Verification items for the finished model (mm, model axes). Round coordinates to 2 decimals unless told otherwise and drop trailing zeros. Order: outer loops, then holes, each group sorted by start corner. A loop starts at its lowest first (then second) coordinate and runs counter-clockwise, first axis right, second up. Notation, with made-up numbers: (-4.5, 32) -> (18.5, 32) arc R23 cw to (18.5, 48) -> close; hole circle Ø5 at (-35.75, 28). An arc over 180 degrees is marked (long way). Put each result on its own line as item: value.
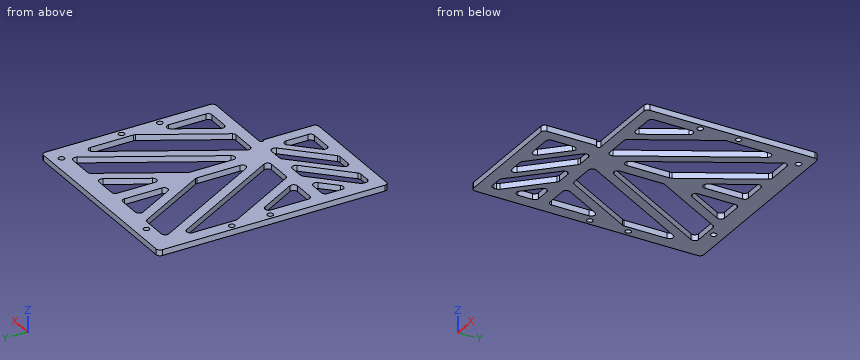
```python
from build123d import *

# Parameters (mm, degrees)
SKETCH_1_W          = 103.5
SKETCH_1_H          = 90
EXTRUDE_1_DEPTH     = 1.5
SKETCH_2_W          = 63.5
SKETCH_2_H          = 30
EXTRUDE_2_DEPTH     = 3
SKETCH_3_R          = 1.05
CUT_EXTRUDE_1_DEPTH = 3
SKETCH_4_R          = 1.525
CUT_EXTRUDE_2_DEPTH = 10
SKETCH_5_R          = 1.525
CUT_EXTRUDE_3_DEPTH = 10
FILLET_1_R          = 2
CUT_EXTRUDE_4_DEPTH = 10
CUT_EXTRUDE_5_DEPTH = 10
FILLET_2_R          = 2


with BuildPart() as part:
    # 草图1 → 凸台-拉伸1 (new, symmetric)
    with BuildSketch(Plane.XY):
        Rectangle(SKETCH_1_W, SKETCH_1_H)
    extrude(amount=EXTRUDE_1_DEPTH, both=True)

    # 草图2 → 凸台-拉伸2 (add)
    with BuildSketch(Plane.XY.offset(1.5)):
        with Locations((-20, -60)):
            Rectangle(SKETCH_2_W, SKETCH_2_H)
    extrude(amount=-EXTRUDE_2_DEPTH)

    # 草图3 → 切除-拉伸1 (cut)
    with BuildSketch(Plane(origin=(0, 0, -1.5), x_dir=(-1, 0, 0), z_dir=(0, 0, -1))):
        with Locations((-11.75, -46.05)):
            Circle(SKETCH_3_R)
    extrude(amount=-CUT_EXTRUDE_1_DEPTH, mode=Mode.SUBTRACT)

    # 草图4 → 切除-拉伸2 (cut)
    with BuildSketch(Plane.XY.offset(1.5)):
        with Locations((-31.749999997, 39.499993227)):
            Circle(SKETCH_4_R)
        with Locations((43.25, 39.499993227)):
            Circle(SKETCH_4_R)
    extrude(amount=-CUT_EXTRUDE_2_DEPTH, mode=Mode.SUBTRACT)

    # 草图5 → 切除-拉伸3 (cut)
    with BuildSketch(Plane(origin=(0, 0, -1.5), x_dir=(-1, 0, 0), z_dir=(0, 0, -1))):
        with Locations((48.75, -15)):
            Circle(SKETCH_5_R)
        with Locations((48.75, 5)):
            Circle(SKETCH_5_R)
    cut_extrude_3 = extrude(amount=-CUT_EXTRUDE_3_DEPTH, mode=Mode.SUBTRACT)

    # 镜向1: 切除-拉伸3 across plane
    add(cut_extrude_3.mirror(Plane(origin=(0, 0, 0), x_dir=(0, 0, 1), z_dir=(1, 0, 0))), mode=Mode.SUBTRACT)

    # 圆角1
    fillet_1_edges = [part.edges().sort_by_distance(p)[0] for p in [
        (11.75, -75, 0),
        (-51.75, -75, 0),
        (51.75, -45, 0),
        (-51.75, 45, 0),
        (51.75, 45, 0),
    ]]
    fillet(fillet_1_edges, radius=FILLET_1_R)

    # 草图6 → 切除-拉伸4 (cut)
    with BuildSketch(Plane(origin=(0, 0, -1.5), x_dir=(-1, 0, 0), z_dir=(0, 0, -1))):
        Polygon((-28.82451653, -39), (-45.25, -9.842339669), (-45.25, -39), align=None)
        Polygon((-5.869390726, -39), (-45.25, 30.906400683), (-45.25, 0.344845419), (-23.085735079, -39), align=None)
        Polygon((-25.164264921, 35.999993227), (-42.380609274, 35.999993227), (-3, -33.906407456), (-3, -3.344852192), align=None)
        Polygon((-3, 35.999993227), (-19.42548347, 35.999993227), (-3, 6.842332896), align=None)
        Polygon((3, 6.842332896), (19.42548347, 35.999993227), (3, 35.999993227), align=None)
        Polygon((42.380609274, 35.999993227), (25.164264921, 35.999993227), (3, -3.344852192), (3, -33.906407456), align=None)
        Polygon((45.25, 0.344845419), (45.25, 30.906400683), (5.869390726, -39), (23.085735079, -39), align=None)
        Polygon((45.25, -39), (45.25, -9.842339669), (28.82451653, -39), align=None)
    extrude(amount=-CUT_EXTRUDE_4_DEPTH, mode=Mode.SUBTRACT)

    # 草图7 → 切除-拉伸5 (cut)
    with BuildSketch(Plane(origin=(0, 0, -1.5), x_dir=(-1, 0, 0), z_dir=(0, 0, -1))):
        Polygon((12.593145751, -69), (-5.75, -50.656854249), (-5.75, -69), align=None)
        Polygon((6.977922061, -45), (-5.75, -45), (18.25, -69), (30.977922061, -69), align=None)
        Polygon((25.362698372, -45), (12.634776311, -45), (36.634776311, -69), (45.25, -69), (45.25, -64.887301628), align=None)
        Polygon((45.25, -45), (31.019552622, -45), (45.25, -59.230447378), align=None)
    extrude(amount=-CUT_EXTRUDE_5_DEPTH, mode=Mode.SUBTRACT)

    # 圆角2
    fillet_2_edges = [part.edges().sort_by_distance(p)[0] for p in [
        (-3, 6.842332896, 0),
        (-3, 35.999993227, 0),
        (-19.42548347, 35.999993227, 0),
        (19.42548347, 35.999993227, 0),
        (3, 35.999993227, 0),
        (3, 6.842332896, 0),
        (45.25, 0.344845419, 0),
        (45.25, 30.906400683, 0),
        (5.869390726, -39, 0),
        (23.085735079, -39, 0),
        (25.164264921, 35.999993227, 0),
        (3, -3.344852192, 0),
        (3, -33.906407456, 0),
        (42.380609274, 35.999993227, 0),
        (-45.25, -9.842339669, 0),
        (-45.25, -39, 0),
        (-28.82451653, -39, 0),
        (-3, -33.906407456, 0),
        (-3, -3.344852192, 0),
        (-25.164264921, 35.999993227, 0),
        (-42.380609274, 35.999993227, 0),
        (-45.25, 30.906400683, 0),
        (-45.25, 0.344845419, 0),
        (-23.085735079, -39, 0),
        (-5.869390726, -39, 0),
        (45.25, -9.842339669, 0),
        (28.82451653, -39, 0),
        (45.25, -39, 0),
        (-25.362698372, -45, 0),
        (-45.25, -64.887301628, 0),
        (-45.25, -69, 0),
        (-36.634776311, -69, 0),
        (-12.634776311, -45, 0),
        (-6.977922061, -45, 0),
        (-30.977922061, -69, 0),
        (-18.25, -69, 0),
        (5.75, -45, 0),
        (-31.019552622, -45, 0),
        (-45.25, -45, 0),
        (-45.25, -59.230447378, 0),
        (5.75, -50.656854249, 0),
        (-12.593145751, -69, 0),
        (5.75, -69, 0),
    ]]
    fillet(fillet_2_edges, radius=FILLET_2_R)


solid = part.part
```
Item 1: Sectioned sample at C-C, the plane y = 28. Record the boundary of the cut face in (x, z), then the cut area to 3 significant figures.
Geometry check:
outline: (-51.75, -1.5) -> (-37.87, -1.5) -> (-37.87, 1.5) -> (-51.75, 1.5) -> close; (-20.66, -1.5) -> (-14.92, -1.5) -> (-14.92, 1.5) -> (-20.66, 1.5) -> close; (-3, -1.5) -> (3, -1.5) -> (3, 1.5) -> (-3, 1.5) -> close; (14.92, -1.5) -> (20.66, -1.5) -> (20.66, 1.5) -> (14.92, 1.5) -> close; (37.87, -1.5) -> (51.75, -1.5) -> (51.75, 1.5) -> (37.87, 1.5) -> close
area: 136 mm2
Item 2: Depth check by flat-ended pin: pin 1 Ø2.5 at (x, y) = (43.25, 39.5) entering from +Z; pin 2 Ø1 at (y, z) = (-59, -1) entering from +X. Enter the tip coordinate at first touch or a pass-through.
Geometry check:
pin 1: through
pin 2: x = 11.75
Item 3: Sectioned sample at D-D, the plane y = 5. Record the boundary of the cut face in (x, z) (3 decimals), then the cut area to 3 significant figures.
Geometry check:
outline: (-51.75, -1.5) -> (-50.275, -1.5) -> (-50.275, 1.5) -> (-51.75, 1.5) -> close; (-47.225, -1.5) -> (-45.25, -1.5) -> (-45.25, 1.5) -> (-47.225, 1.5) -> close; (-30.656, -1.5) -> (-24.917, -1.5) -> (-24.917, 1.5) -> (-30.656, 1.5) -> close; (-7.701, -1.5) -> (7.701, -1.5) -> (7.701, 1.5) -> (-7.701, 1.5) -> close; (24.917, -1.5) -> (30.656, -1.5) -> (30.656, 1.5) -> (24.917, 1.5) -> close; (45.25, -1.5) -> (47.225, -1.5) -> (47.225, 1.5) -> (45.25, 1.5) -> close; (50.275, -1.5) -> (51.75, -1.5) -> (51.75, 1.5) -> (50.275, 1.5) -> close
area: 101 mm2
Item 4: Sectioned sample at A-A, the plane y = -25. Record the boundary of the cut face in (x, z).
Geometry check:
outline: (-51.75, -1.5) -> (-45.25, -1.5) -> (-45.25, 1.5) -> (-51.75, 1.5) -> close; (-36.71, -1.5) -> (-30.97, -1.5) -> (-30.97, 1.5) -> (-36.71, 1.5) -> close; (-13.76, -1.5) -> (-8.02, -1.5) -> (-8.02, 1.5) -> (-13.76, 1.5) -> close; (-3, -1.5) -> (3, -1.5) -> (3, 1.5) -> (-3, 1.5) -> close; (8.02, -1.5) -> (13.76, -1.5) -> (13.76, 1.5) -> (8.02, 1.5) -> close; (30.97, -1.5) -> (36.71, -1.5) -> (36.71, 1.5) -> (30.97, 1.5) -> close; (45.25, -1.5) -> (51.75, -1.5) -> (51.75, 1.5) -> (45.25, 1.5) -> close
Item 5: Material ranges on line 1 along Y through (x, z) = (48.75, -0.7) (3 decimals); line 2 along Y through (x, z) = (-48.75, -0.85) (3 decimals); line 3 along X through (y, z) = (-10, 0.1), recorded low to high.
Geometry check:
line 1: -45 to -16.525, -13.475 to 3.475, 6.525 to 45
line 2: -75 to -16.525, -13.475 to 3.475, 6.525 to 45
line 3: -51.75 to -39.42, -22.21 to -16.47, -3 to 3, 16.47 to 22.21, 39.42 to 51.75
Item 6: Sectioned sample at B-B, the plane z = 0.45. Give the number of separate pieces and of enclosed holes in the cut face, then the cut area to 3 significant figures.
Geometry check:
separate pieces: 1
enclosed holes: 18
area: 5,720 mm2
